```python
from build123d import *

# Parameters (mm, degrees)
EXTRUDE_1_DEPTH      = 2
EXTRUDE_2_DEPTH      = 29
EXTRUDE_2_DEPTH_BACK = 2
CUT_EXTRUDE_5_REACH  = 60.965
SKETCH_3_R           = 0.75
SKETCH_3_W           = 9
SKETCH_3_H           = 20.1
CUT_EXTRUDE_7_REACH  = 61.851
SKETCH_12_R          = 0.75
SKETCH_12_W          = 9
SKETCH_12_H          = 20.1
CUT_EXTRUDE_8_REACH  = 71.217
SKETCH_13_R          = 1
SKETCH_13_W          = 16
SKETCH_13_H          = 38.074491789
SKETCH_13_W_2        = 2
SKETCH_13_H_2        = 3
CHAMFER_4_SIZE       = 1
CHAMFER_5_SIZE       = 2
EXTRUDE_START        = -29
SKETCH_14_W          = 3
SKETCH_14_H          = 6
SKETCH_14_W_2        = 4.936896873
SKETCH_14_H_2        = 2.5
EXTRUDE_8_DEPTH      = 29
CHAMFER_6_SIZE       = 2
EXTRUDE_START_2      = 3
SKETCH_15_R          = 2
SKETCH_15_R_2        = 1
EXTRUDE_9_DEPTH      = 3
CUT_EXTRUDE_9_REACH  = 60.599
SKETCH_16_W          = 3
SKETCH_16_H          = 20
EXTRUDE_10_DEPTH     = 2
EXTRUDE_11_DEPTH     = 24.1
CUT_EXTRUDE_11_REACH = 71.217
SKETCH_20_W          = 33.566306147
SKETCH_20_H          = 6.687524296


with BuildPart() as part:
    # 草圖1 → 填料-伸長1 (new body)
    with BuildSketch(Plane.XY):
        Polygon((-15, 0), (15, 0), (15, -1), (18.708735418, -10.179442277), (15, -11.67786865), (15, -60), (-15, -60), (-15, -11.67786865), (-18.708735418, -10.179442277), (-15, -1), align=None)
    extrude(amount=EXTRUDE_1_DEPTH)

    # 草圖2 → 填料-伸長2 (add, two sides: drawn at the far end of the back side and taken through both)
    with BuildSketch(Plane.XY.offset(2).offset(-EXTRUDE_2_DEPTH_BACK)):
        Polygon((-18.708735418, -10.179442277), (-9.436896873, -13.925508211), (9.436896873, -13.925508211), (18.708735418, -10.179442277), (17.584915638, -7.397890713), (8.313077092, -11.143956647), (-8.313077092, -11.143956647), (-17.584915638, -7.397890713), align=None)
    extrude(amount=EXTRUDE_2_DEPTH + EXTRUDE_2_DEPTH_BACK)

    # 草圖3 → 除料-伸長5 (cut, up to next)
    with BuildSketch(Plane(origin=(4.914686172, -15.752599933, 0), x_dir=(0.9271838545667884, 0.37460659341590963, 0), z_dir=(-0.37460659341590963, 0.9271838545667884, 0)), mode=Mode.PRIVATE) as cut_extrude_5_sk1:
        with Locations(Location((10.377361354, -5.2, 0), (0, 0, 180))):
            Circle(SKETCH_3_R)
    cut_extrude_5_tool1 = extrude(cut_extrude_5_sk1.sketch, amount=CUT_EXTRUDE_5_REACH, mode=Mode.PRIVATE) & part.part
    # 草圖3 → 除料-伸長5 (cut, up to next)
    with BuildSketch(Plane(origin=(4.914686172, -15.752599933, 0), x_dir=(0.9271838545667884, 0.37460659341590963, 0), z_dir=(-0.37460659341590963, 0.9271838545667884, 0)), mode=Mode.PRIVATE) as cut_extrude_5_sk2:
        with Locations(Location((10.377361354, -28.7, 0), (0, 0, 180))):
            Circle(SKETCH_3_R)
    cut_extrude_5_tool2 = extrude(cut_extrude_5_sk2.sketch, amount=CUT_EXTRUDE_5_REACH, mode=Mode.PRIVATE) & part.part
    # 草圖3 → 除料-伸長5 (cut, up to next)
    with BuildSketch(Plane(origin=(4.914686172, -15.752599933, 0), x_dir=(0.9271838545667884, 0.37460659341590963, 0), z_dir=(-0.37460659341590963, 0.9271838545667884, 0)), mode=Mode.PRIVATE) as cut_extrude_5_sk3:
        with Locations((10.377361354, -16.95)):
            Rectangle(SKETCH_3_W, SKETCH_3_H)
    cut_extrude_5_tool3 = extrude(cut_extrude_5_sk3.sketch, amount=CUT_EXTRUDE_5_REACH, mode=Mode.PRIVATE) & part.part
    add(cut_extrude_5_tool1.solids().sort_by_distance((14.536408, -11.865172, 5.2))[0], mode=Mode.SUBTRACT)
    add(cut_extrude_5_tool2.solids().sort_by_distance((14.536408, -11.865172, 28.7))[0], mode=Mode.SUBTRACT)
    add(cut_extrude_5_tool3.solids().sort_by_distance((14.536408, -11.865172, 16.95))[0], mode=Mode.SUBTRACT)

    # 草圖12 → 除料-伸長7 (cut, up to next)
    with BuildSketch(Plane(origin=(-6.161016101, -15.249049955, 0), x_dir=(0.9271838545667846, -0.3746065934159192, 0), z_dir=(-0.3746065934159192, -0.9271838545667846, 0)), mode=Mode.PRIVATE) as cut_extrude_7_sk1:
        with Locations((-9.033151225, 28.7)):
            Circle(SKETCH_12_R)
    cut_extrude_7_tool1 = extrude(cut_extrude_7_sk1.sketch, amount=-CUT_EXTRUDE_7_REACH, mode=Mode.PRIVATE) & part.part
    # 草圖12 → 除料-伸長7 (cut, up to next)
    with BuildSketch(Plane(origin=(-6.161016101, -15.249049955, 0), x_dir=(0.9271838545667846, -0.3746065934159192, 0), z_dir=(-0.3746065934159192, -0.9271838545667846, 0)), mode=Mode.PRIVATE) as cut_extrude_7_sk2:
        with Locations((-9.033151225, 5.2)):
            Circle(SKETCH_12_R)
    cut_extrude_7_tool2 = extrude(cut_extrude_7_sk2.sketch, amount=-CUT_EXTRUDE_7_REACH, mode=Mode.PRIVATE) & part.part
    # 草圖12 → 除料-伸長7 (cut, up to next)
    with BuildSketch(Plane(origin=(-6.161016101, -15.249049955, 0), x_dir=(0.9271838545667846, -0.3746065934159192, 0), z_dir=(-0.3746065934159192, -0.9271838545667846, 0)), mode=Mode.PRIVATE) as cut_extrude_7_sk3:
        with Locations((-9.033151225, 16.95)):
            Rectangle(SKETCH_12_W, SKETCH_12_H)
    cut_extrude_7_tool3 = extrude(cut_extrude_7_sk3.sketch, amount=-CUT_EXTRUDE_7_REACH, mode=Mode.PRIVATE) & part.part
    add(cut_extrude_7_tool1.solids().sort_by_distance((-14.536408, -11.865172, 28.7))[0], mode=Mode.SUBTRACT)
    add(cut_extrude_7_tool2.solids().sort_by_distance((-14.536408, -11.865172, 5.2))[0], mode=Mode.SUBTRACT)
    add(cut_extrude_7_tool3.solids().sort_by_distance((-14.536408, -11.865172, 16.95))[0], mode=Mode.SUBTRACT)

    # 草圖13 → 除料-伸長8 (cut, up to next)
    with BuildSketch(Plane.XY.offset(2), mode=Mode.PRIVATE) as cut_extrude_8_sk1:
        with Locations((-13, -30)):
            Circle(SKETCH_13_R)
    cut_extrude_8_tool1 = extrude(cut_extrude_8_sk1.sketch, amount=-CUT_EXTRUDE_8_REACH, mode=Mode.PRIVATE) & part.part
    # 草圖13 → 除料-伸長8 (cut, up to next)
    with BuildSketch(Plane.XY.offset(2), mode=Mode.PRIVATE) as cut_extrude_8_sk2:
        with Locations((13, -30)):
            Circle(SKETCH_13_R)
    cut_extrude_8_tool2 = extrude(cut_extrude_8_sk2.sketch, amount=-CUT_EXTRUDE_8_REACH, mode=Mode.PRIVATE) & part.part
    # 草圖13 → 除料-伸長8 (cut, up to next)
    with BuildSketch(Plane.XY.offset(2), mode=Mode.PRIVATE) as cut_extrude_8_sk3:
        with Locations((-13, -57.5)):
            Circle(SKETCH_13_R)
    cut_extrude_8_tool3 = extrude(cut_extrude_8_sk3.sketch, amount=-CUT_EXTRUDE_8_REACH, mode=Mode.PRIVATE) & part.part
    # 草圖13 → 除料-伸長8 (cut, up to next)
    with BuildSketch(Plane.XY.offset(2), mode=Mode.PRIVATE) as cut_extrude_8_sk4:
        with Locations((13, -57.5)):
            Circle(SKETCH_13_R)
    cut_extrude_8_tool4 = extrude(cut_extrude_8_sk4.sketch, amount=-CUT_EXTRUDE_8_REACH, mode=Mode.PRIVATE) & part.part
    # 草圖13 → 除料-伸長8 (cut, up to next)
    with BuildSketch(Plane.XY.offset(2), mode=Mode.PRIVATE) as cut_extrude_8_sk5:
        with Locations((0, -37.962754105)):
            Rectangle(SKETCH_13_W, SKETCH_13_H)
    cut_extrude_8_tool5 = extrude(cut_extrude_8_sk5.sketch, amount=-CUT_EXTRUDE_8_REACH, mode=Mode.PRIVATE) & part.part
    # 草圖13 → 除料-伸長8 (cut, up to next)
    with BuildSketch(Plane.XY.offset(2), mode=Mode.PRIVATE) as cut_extrude_8_sk6:
        with Locations((-14, -43.5)):
            Rectangle(SKETCH_13_W_2, SKETCH_13_H_2)
    cut_extrude_8_tool6 = extrude(cut_extrude_8_sk6.sketch, amount=-CUT_EXTRUDE_8_REACH, mode=Mode.PRIVATE) & part.part
    # 草圖13 → 除料-伸長8 (cut, up to next)
    with BuildSketch(Plane.XY.offset(2), mode=Mode.PRIVATE) as cut_extrude_8_sk7:
        with Locations((14, -43.5)):
            Rectangle(SKETCH_13_W_2, SKETCH_13_H_2)
    cut_extrude_8_tool7 = extrude(cut_extrude_8_sk7.sketch, amount=-CUT_EXTRUDE_8_REACH, mode=Mode.PRIVATE) & part.part
    add(cut_extrude_8_tool1.solids().sort_by_distance((-13, -30, 2))[0], mode=Mode.SUBTRACT)
    add(cut_extrude_8_tool2.solids().sort_by_distance((13, -30, 2))[0], mode=Mode.SUBTRACT)
    add(cut_extrude_8_tool3.solids().sort_by_distance((-13, -57.5, 2))[0], mode=Mode.SUBTRACT)
    add(cut_extrude_8_tool4.solids().sort_by_distance((13, -57.5, 2))[0], mode=Mode.SUBTRACT)
    add(cut_extrude_8_tool5.solids().sort_by_distance((0, -37.962754, 2))[0], mode=Mode.SUBTRACT)
    add(cut_extrude_8_tool6.solids().sort_by_distance((-14, -43.5, 2))[0], mode=Mode.SUBTRACT)
    add(cut_extrude_8_tool7.solids().sort_by_distance((14, -43.5, 2))[0], mode=Mode.SUBTRACT)

    # 導角4
    chamfer_4_edges = [part.edges().sort_by_distance(p)[0] for p in [
        (-15, 0, 1),
        (15, 0, 1),
    ]]
    chamfer(chamfer_4_edges, length=CHAMFER_4_SIZE - 0.0001)  # a hair under: the kernel refuses the full size

    # 導角5
    chamfer_5_edges = [part.edges().sort_by_distance(p)[0] for p in [
        (-12.948996365, -9.27092368, 2),
        (0, -11.143956647, 2),
        (12.948996365, -9.27092368, 2),
    ]]
    chamfer(chamfer_5_edges, length=CHAMFER_5_SIZE)

    # 草圖14 → 填料-伸長8 (add)
    with BuildSketch(Plane.XY.offset(31).offset(EXTRUDE_START)):
        with Locations((0, -13.425508211)):
            Rectangle(SKETCH_14_W, SKETCH_14_H)
        with Locations((-6.968448437, -15.175508211)):
            Rectangle(SKETCH_14_W_2, SKETCH_14_H_2)
        with Locations((6.968448437, -15.175508211)):
            Rectangle(SKETCH_14_W_2, SKETCH_14_H_2)
    extrude(amount=EXTRUDE_8_DEPTH)

    # 導角6
    chamfer_6_edges = [part.edges().sort_by_distance(p)[0] for p in [
        (0, -16.425508211, 31),
        (-6.968448436, -16.425508211, 31),
        (6.968448436, -16.425508211, 31),
    ]]
    chamfer(chamfer_6_edges, length=CHAMFER_6_SIZE)

    # 草圖15 → 填料-伸長9 (add)
    # profile 1 of 4: a face of its own
    with BuildSketch(Plane.XY.offset(2).offset(EXTRUDE_START_2)):
        with Locations(Location((-13, -30, 0), (0, 0, 180))):
            Circle(SKETCH_15_R)
        with Locations((-13, -30)):
            Circle(SKETCH_15_R_2, mode=Mode.SUBTRACT)
    # profile 2 of 4: a face of its own
    with BuildSketch(Plane.XY.offset(2).offset(EXTRUDE_START_2)):
        with Locations((13, -30)):
            Circle(SKETCH_15_R)
        with Locations((13, -30)):
            Circle(SKETCH_15_R_2, mode=Mode.SUBTRACT)
    # profile 3 of 4: a face of its own
    with BuildSketch(Plane.XY.offset(2).offset(EXTRUDE_START_2)):
        with Locations((13, -57.5)):
            Circle(SKETCH_15_R)
        with Locations((13, -57.5)):
            Circle(SKETCH_15_R_2, mode=Mode.SUBTRACT)
    # profile 4 of 4: a face of its own
    with BuildSketch(Plane.XY.offset(2).offset(EXTRUDE_START_2)):
        with Locations(Location((-13, -57.5, 0), (0, 0, 180))):
            Circle(SKETCH_15_R)
        with Locations((-13, -57.5)):
            Circle(SKETCH_15_R_2, mode=Mode.SUBTRACT)
    extrude(amount=-EXTRUDE_9_DEPTH)

    # 草圖16 → 除料-伸長9 (cut, up to next)
    with BuildSketch(Plane.XZ.offset(13.925508211), mode=Mode.PRIVATE) as cut_extrude_9_sk1:
        with Locations((-3, 15)):
            Rectangle(SKETCH_16_W, SKETCH_16_H)
    cut_extrude_9_tool1 = extrude(cut_extrude_9_sk1.sketch, amount=-CUT_EXTRUDE_9_REACH, mode=Mode.PRIVATE) & part.part
    # 草圖16 → 除料-伸長9 (cut, up to next)
    with BuildSketch(Plane.XZ.offset(13.925508211), mode=Mode.PRIVATE) as cut_extrude_9_sk2:
        with Locations((3, 15)):
            Rectangle(SKETCH_16_W, SKETCH_16_H)
    cut_extrude_9_tool2 = extrude(cut_extrude_9_sk2.sketch, amount=-CUT_EXTRUDE_9_REACH, mode=Mode.PRIVATE) & part.part
    add(cut_extrude_9_tool1.solids().sort_by_distance((-3, -13.925508, 15))[0], mode=Mode.SUBTRACT)
    add(cut_extrude_9_tool2.solids().sort_by_distance((3, -13.925508, 15))[0], mode=Mode.SUBTRACT)

    # 草圖17 → 填料-伸長10 (add)
    with BuildSketch(Plane(origin=(0, 0, 0), x_dir=(-1, 0, 0), z_dir=(0, 0, -1))):
        Polygon((-18.708735418, -10.179442277), (-15, -19.67786865), (-15, -11.67786865), align=None)
        Polygon((18.708735418, -10.179442277), (15, -11.67786865), (15, -19.67786865), align=None)
    extrude(amount=-EXTRUDE_10_DEPTH)

    # 草圖18 → 填料-伸長11 (add)
    with BuildSketch(Plane.XY.offset(31)):
        Polygon((-17.584915638, -7.397890713), (-18.708735418, -10.179442277), (-18.152425106, -10.404206233), (-17.028605325, -7.622654669), align=None)
        Polygon((17.584915638, -7.397890713), (18.708735418, -10.179442277), (18.152425106, -10.404206233), (17.028605325, -7.622654669), align=None)
    extrude(amount=-EXTRUDE_11_DEPTH)

    # 草圖20 → 除料-伸長11 (cut, up to next)
    with BuildSketch(Plane.XY.offset(2), mode=Mode.PRIVATE) as cut_extrude_11_sk1:
        with Locations((-0.052549378, -2.199760856)):
            Rectangle(SKETCH_20_W, SKETCH_20_H)
    cut_extrude_11_tool1 = extrude(cut_extrude_11_sk1.sketch, amount=-CUT_EXTRUDE_11_REACH, mode=Mode.PRIVATE) & part.part
    add(cut_extrude_11_tool1.solids().sort_by_distance((-0.052549, -2.199761, 2))[0], mode=Mode.SUBTRACT)


solid = part.part
```
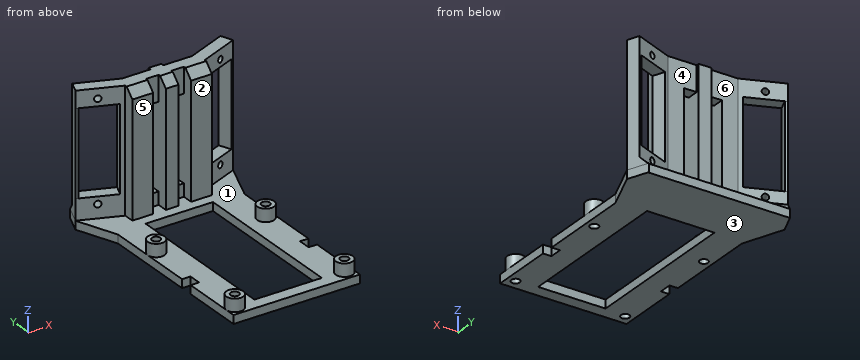
Work out the finished part from the listing and answer in its coordinate system (mm). Face numbers are marked on the shaded views. A direction names the side the tool comes from. Give positions to 0.01 mm unless a question says otherwise; leave off trailing zeros. Loops run counter-clockwise (first coordinate to the right, second up) from the corner with the lowest first, then second, coordinate; pieces in that order, holes last. Notation, with made-up numbers: (79.5, 8) - (99.5, 8) arc R30 cw to (99.5, 40) - close; hole circle Ø2 at (83.25, 34). An arc over 180 degrees is marked (long way). Use CSV: the item, a comma, the result in double quotes. Start each with the question number.
(1) Determine the mould class of the marked faces 4, 5 and 6 for opening direction X: released by +X, released by -X, zero draft, split by the parting line, or undercut.
(2) A tool of negligible diameter and unlimited length cuts with its end or side. For the marked faces 1, 2 and 3, from which of +Z, -Z, +X, -X, +Y, -Y can it reach the whole face along a straight path? Write none if from no direction.
(3) Each of these flat-tipped pins is pushed along its axis until it touches: pin 1 (1 mm diameter, centred on x = 13.5, z = 0.5, fed in from +Y); pin 2 (1.2 mm diameter, centred on x = -1.5, y = -7.5, fed in from +Z); pin 3 (2.5 mm diameter, centred on x = 13, y = -57.5, fed in from -Z); pin 4 (2.5 mm diameter, centred on x = -0.5, z = 11, fed in from +Y). Where does it stop, or does it pass through?
(4) Find section A-A, the plane y = -37. Determine the outline of the cut face in (x, z), plus the area to 3 significant figures.
(5) Find the intervals of material crossed by L1, parallel to Y at x = 13, z = 3.3; L2, parallel to Z at x = 11, y = -30.5; L3, parallel to Y at x = -13, z = 4.5, in increasing order.
(6) Find section B-B, the plane z = 23.5. Determine the outline of the cut face in (x, y).
Results found:
1,face 4,"undercut"
1,face 5,"zero draft"
1,face 6,"undercut"
2,face 1,"+Z"
2,face 2,"+Z, +X, -X, -Y"
2,face 3,"-Z, +X, -X, +Y, -Y"
3,pin 1,"y = -5.54"
3,pin 2,"z = 2"
3,pin 3,"z = 0"
3,pin 4,"y = -10.43"
4,outline,"(-15, 0) - (-8, 0) - (-8, 2) - (-15, 2) - close; (8, 0) - (15, 0) - (15, 2) - (8, 2) - close"
4,area,"28.0 mm^2"
5,L1,"-59.5 to -58.5, -56.5 to -55.5, -32 to -31, -29 to -28, -12.49 to -8.5"
5,L2,"0 to 2"
5,L3,"-59.5 to -58.5, -56.5 to -55.5, -32 to -31, -29 to -28, -12.49 to -9.25"
6,outline,"(-18.71, -10.18) - (-18.15, -10.4) - (-17.03, -7.62) - (-17.58, -7.4) - close; (-10.36, -13.55) - (-9.44, -13.93) - (-9.44, -16.43) - (-4.5, -16.43) - (-4.5, -11.14) - (-8.31, -11.14) - (-9.24, -10.77) - close; (-1.5, -16.43) - (1.5, -16.43) - (1.5, -10.43) - (-1.5, -10.43) - close; (4.5, -16.43) - (9.44, -16.43) - (9.44, -13.93) - (10.36, -13.55) - (9.24, -10.77) - (8.31, -11.14) - (4.5, -11.14) - close; (17.03, -7.62) - (18.15, -10.4) - (18.71, -10.18) - (17.58, -7.4) - close"
